from build123d import *

# Parameters (mm, degrees)
CUT_EXTRUDE_1_DEPTH = 2
FILLET_1_R          = 0.3
CHAMFER_1_SIZE      = 0.3


with BuildPart() as part:
    # Эскиз1 → Повернуть1 (revolve)
    with BuildSketch(Plane(origin=(0, 0, 0), x_dir=(0, 0, -1), z_dir=(1, 0, 0))):
        Polygon((0, 0), (0, 2.5), (3, 2.5), (3, 1.5), (28, 1.5), (28, 0), align=None)
    revolve(axis=Axis((0, 0, 0), (0, 0, 1)))

    # Эскиз2 → Вырез-Вытянуть1 (cut)
    with BuildSketch(Plane.XY):
        Polygon((1.443375673, 0), (0.721687836, 1.25), (-0.721687836, 1.25), (-1.443375673, 0), (-0.721687836, -1.25), (0.721687836, -1.25), align=None)
    extrude(amount=-CUT_EXTRUDE_1_DEPTH, mode=Mode.SUBTRACT)

    # Скругление1
    fillet_1_edges = [part.edges().sort_by_distance(p)[0] for p in [
        (0, -1.5, -3),
    ]]
    fillet(fillet_1_edges, radius=FILLET_1_R)

    # Фаска1
    chamfer_1_edges = [part.edges().sort_by_distance(p)[0] for p in [
        (0, -1.5, -28),
    ]]
    chamfer(chamfer_1_edges, length=CHAMFER_1_SIZE)


solid = part.part
Geometry check sheet. Reference: the model listing, model coordinates, mm. A direction names the side the tool comes from. Round coordinates to 2 decimals unless told otherwise and drop trailing zeros. Order: outer loops, then holes, each group sorted by start corner. A loop starts at its lowest first (then second) coordinate and runs counter-clockwise, first axis right, second up. Notation, with made-up numbers: M 80,12 L 111,12 A34 cw 111,44 Z; hole C 17,-26.75 d1. An arc over 180 degrees is marked long. Answer in a Markdown table with one row per item.
(1) Sectioned sample at B-B, the plane z = -8.5. Record the cut outline in (x, y), and give its area (3 significant figures).
Responses:
| item | result |
|---|---|
| outline | C 0,0 d3 |
| area | 7.07 mm² |
(2) Draft check along Y on faces 1 (the face through (0, 0, -28)), 2 (the face through (0, -1.25, -1)), 3 (the face through (2.44, -0.54, -1.52)). Enter one of: released by +Y, released by -Y, zero draft, split by the parting line, or undercut.
Responses:
| item | result |
|---|---|
| face 1 | zero draft |
| face 2 | undercut |
| face 3 | split by the parting line |
(3) Scan lines: probe 1 along Z at (x, y) = (1.35, 1.6); probe 2 along Z at (x, y) = (-0.1, 0.5); probe 3 along Y at (x, z) = (0.05, -15.25). Record each from-to range of solid material in increasing order. Write a range as from..to.
Responses:
| item | result |
|---|---|
| probe 1 | z = -3..0 |
| probe 2 | z = -28..-2 |
| probe 3 | y = -1.5..1.5 |
(4) Tool access check on faces 4 (the face through (1.08, -0.63, -0.99)), 5 (the face through (1.1, -1.1, 0)), 6 (the face through (-0.07, -1.5, -15.67)). Record the directions out of +Z, -Z, +X, -X, +Y, -Y that give a thin tool (end or side, any length) a straight path to the whole face; none if there is none.
Responses:
| item | result |
|---|---|
| face 4 | +Z |
| face 5 | +Z, +X, -X, +Y, -Y |
| face 6 | -Z |
(5) Sectioned sample at A-A, the plane x = 0. Record the cut outline in (y, z).
Responses:
| item | result |
|---|---|
| outline | M -2.5,-3 L -1.8,-3 A0.3 cw -1.5,-3.3 L -1.5,-27.7 L -1.2,-28 L 1.2,-28 L 1.5,-27.7 L 1.5,-3.3 A0.3 cw 1.8,-3 L 2.5,-3 L 2.5,0 L 1.25,0 L 1.25,-2 L -1.25,-2 L -1.25,0 L -2.5,0 Z |
(6) Go/stop test with flat-tipped pins: P1, Ø2, axis at x = 1, z = -11.5, coming from the +Y side; P2, Ø3, axis at x = -0.5, y = -0.5, coming from the +Z side; P3, Ø3, axis at x = 2, y = -2, coming from the -Z side; P4, Ø1.5, axis at x = 1.5, z = -22.5, coming from the +Y side. Record where each tip stops, or that it passes through.
Responses:
| item | result |
|---|---|
| P1 | stops at y = 1.5 |
| P2 | stops at z = 0 |
| P3 | stops at z = -27.87 |
| P4 | stops at y = 1.3 |
